Can you work these out from the drawing? Everything is in mm from the part's minimum corner. Coordinates: 2 decimals unless noted, no trailing zeros. Write each loop counter-clockwise with the first axis right and the second up, starting at its lowest first coordinate (ties: lowest second). Pieces come first, ordered by that corner, then holes. Notation, with made-up numbers: (4, 67) -> (28, 67) arc R23 ccw to (28, 76) -> close; hole circle Ø10 at (23, 51). An arc over 180 degrees is marked (long way). Use a Markdown table: item, result. Add a question column.
Item 1: Imagine slicing it at D-D, the plane x = 12.2. Write out the boundary of the cut face in (y, z).
Item 2: If I drill on line 1 along Z through (x, y) = (42.2, 1.5); line 2 along Y through (x, z) = (37.5, 31.5); line 3 along Z through (x, y) = (12.2, 2), over which ranges is the centre line in solid material (lowest first)? Write a range as from..to.
Item 3: Imagine slicing it at C-C, the plane x = 42.2. Write out the boundary of the cut face in (y, z) (1 decimal).
Item 4: Imagine slicing it at B-B, the plane y = 1.55. Write out the boundary of the cut face in (x, z).
Item 5: Will this pin go through, and if not, where does the flat tip stop? pin 1 Ø12 at (x, z) = (29.5, 25.5) entering from -Y.
Item 6: Imagine slicing it at A-A, the plane z = 4. Write out the boundary of the cut face in (x, y), and give its area (3 significant figures).
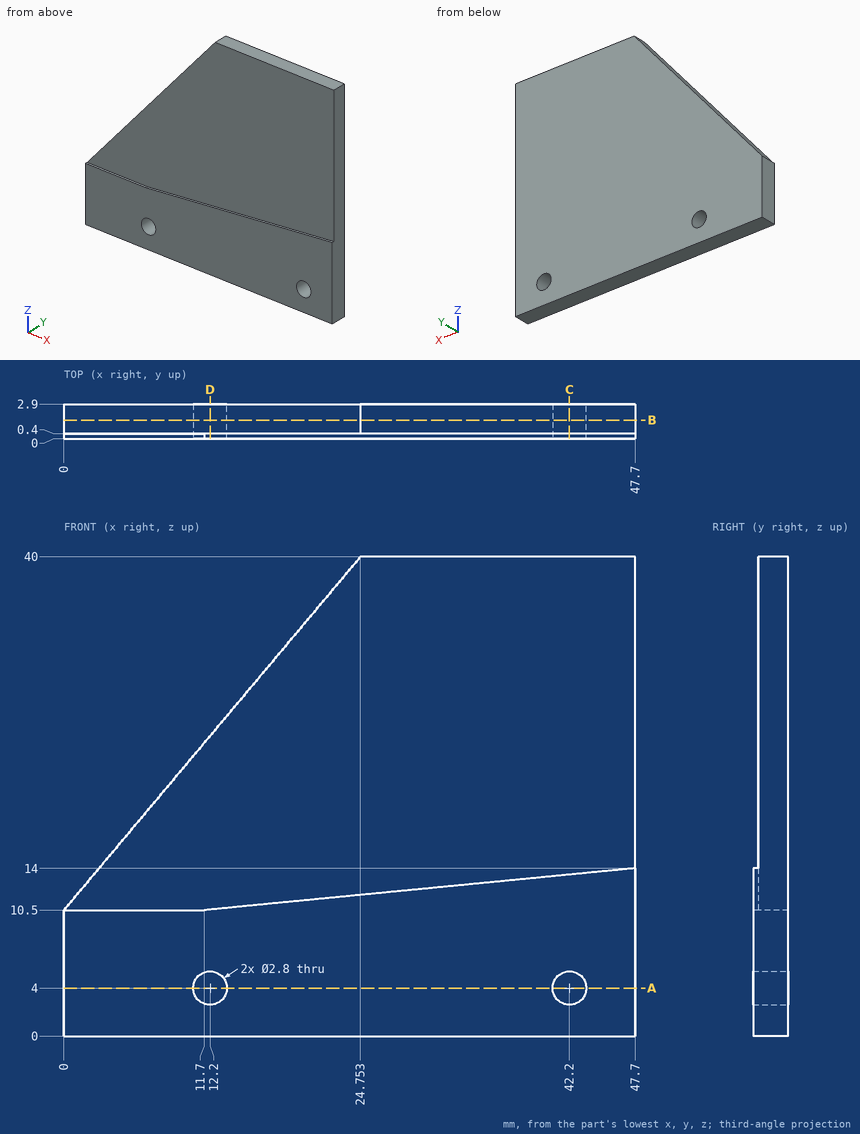
Ans:
| question | item | result |
|---|---|---|
| 1 | outline | (0, 0) -> (2.9, 0) -> (2.9, 2.6) -> (0, 2.6) -> close; (0, 5.4) -> (2.9, 5.4) -> (2.9, 25.04) -> (0.4, 25.04) -> (0.4, 10.55) -> (0, 10.55) -> close |
| 2 | line 1 | z = 0..2.6, 5.4..40 |
| 2 | line 2 | y = 0.4..2.9 |
| 2 | line 3 | z = 0..2.6, 5.4..25.04 |
| 3 | outline | (0, 0) -> (2.9, 0) -> (2.9, 2.6) -> (0, 2.6) -> close; (0, 5.4) -> (2.9, 5.4) -> (2.9, 40) -> (0.4, 40) -> (0.4, 13.5) -> (0, 13.5) -> close |
| 4 | outline | (0, 0) -> (47.7, 0) -> (47.7, 40) -> (24.75, 40) -> (0, 10.5) -> close; hole circle Ø2.8 at (12.2, 4); hole circle Ø2.8 at (42.2, 4) |
| 5 | pin 1 | stops at y = 0.4 |
| 6 | outline | (0, 0) -> (10.8, 0) -> (10.8, 2.9) -> (0, 2.9) -> close; (13.6, 0) -> (40.8, 0) -> (40.8, 2.9) -> (13.6, 2.9) -> close; (43.6, 0) -> (47.7, 0) -> (47.7, 2.9) -> (43.6, 2.9) -> close |
| 6 | area | 122 mm^2 |
